Source: CAD feature listing. Evaluate the final solid. Frame: model axes, mm. Face numbers are marked on the shaded views. A direction names the side the tool comes from. Coordinates: 2 decimals unless noted, no trailing zeros. Order: outer loops, then holes, each group sorted by start corner. A loop starts at its lowest first (then second) coordinate and runs counter-clockwise, first axis right, second up. Notation, with made-up numbers: (84, 55) -> (103, 55) arc R19 cw to (103, 88) -> close; hole circle Ø7 at (73, 14.25). An arc over 180 degrees is marked (long way). Put each result on its own line as item: value.
from build123d import *

# Parameters (mm, degrees)
BOSS_EXTRUDE1_DEPTH      = 3
SKETCH4_R                = 2
CUT_EXTRUDE1_DEPTH       = 3
SKETCH5_R                = 3
CUT_EXTRUDE2_DEPTH       = 1
SKETCH6_R                = 1.5
CUT_EXTRUDE3_DEPTH       = 2
BOSS_EXTRUDE2_DEPTH      = 40
BOSS_EXTRUDE3_DEPTH      = 30
BOSS_EXTRUDE3_DEPTH_BACK = 30
SKETCH7_R                = 2
CUT_EXTRUDE5_REACH       = 83.646


with BuildPart() as part:
    # Sketch2 → Boss-Extrude1 (new body)
    with BuildSketch(Plane.XY):
        Polygon((33.535533906, -16.035533906), (3.535533906, -16.035533906), (0, -12.5), (0, 12.5), (3.535533906, 16.035533906), (23.535533906, 16.035533906), (56.464466094, 5.07852329), (60, 1.542989384), (60, -8.457010616), (56.464466094, -11.992544522), align=None)
    boss_extrude1 = extrude(amount=BOSS_EXTRUDE1_DEPTH)

    # Sketch4 → Cut-Extrude1 (cut)
    with BuildSketch(Plane(origin=(0, 0, 0), x_dir=(-1, 0, 0), z_dir=(0, 0, -1))):
        with Locations((-18, -1.035533906)):
            Circle(SKETCH4_R)
    cut_extrude1 = extrude(amount=-CUT_EXTRUDE1_DEPTH, mode=Mode.SUBTRACT)

    # Sketch5 → Cut-Extrude2 (cut)
    with BuildSketch(Plane(origin=(0, 0, 0), x_dir=(-1, 0, 0), z_dir=(0, 0, -1))):
        with Locations((-18, 6.964466094)):
            Circle(SKETCH5_R)
        with Locations((-10, -1.035533906)):
            Circle(SKETCH5_R)
        with Locations((-18, -9.035533906)):
            Circle(SKETCH5_R)
        with Locations((-26, -1.035533906)):
            Circle(SKETCH5_R)
    cut_extrude2 = extrude(amount=-CUT_EXTRUDE2_DEPTH, mode=Mode.SUBTRACT)

    # Sketch6 → Cut-Extrude3 (cut)
    with BuildSketch(Plane(origin=(0, 0, 1), x_dir=(-1, 0, 0), z_dir=(0, 0, -1))):
        with Locations((-18, 6.964466094)):
            Circle(SKETCH6_R)
        with Locations((-26, -1.035533906)):
            Circle(SKETCH6_R)
        with Locations((-10, -1.035533906)):
            Circle(SKETCH6_R)
        with Locations((-18, -9.035533906)):
            Circle(SKETCH6_R)
    cut_extrude3 = extrude(amount=-CUT_EXTRUDE3_DEPTH, mode=Mode.SUBTRACT)

    # Sketch3 → Boss-Extrude2 (add)
    with BuildSketch(Plane.XY.offset(3)):
        Polygon((8.69213043, 9.878421931), (7.795554958, 13.224487146), (4.449489743, 14.121062618), (2, 11.671572875), (2.896575472, 8.32550766), (6.242640687, 7.428932188), align=None)
        Polygon((36.226681597, -13.530158735), (37.411474128, -10.27496801), (35.184792531, -7.621312217), (31.773318403, -8.22284715), (30.588525872, -11.478037875), (32.815207469, -14.131693668), align=None)
        Polygon((36.846550019, 6.760383974), (36.24355834, 9.699159405), (33.397008321, 10.646341008), (31.153449981, 8.65474718), (31.75644166, 5.715971749), (34.602991679, 4.768790146), align=None)
    extrude(amount=BOSS_EXTRUDE2_DEPTH)

    # Mirror1: Boss-Extrude1, Cut-Extrude1, Cut-Extrude2, Cut-Extrude3 across plane
    add(boss_extrude1.mirror(Plane.XY.offset(23)))
    add(cut_extrude1.mirror(Plane.XY.offset(23)), mode=Mode.SUBTRACT)
    add(cut_extrude2.mirror(Plane.XY.offset(23)), mode=Mode.SUBTRACT)
    add(cut_extrude3.mirror(Plane.XY.offset(23)), mode=Mode.SUBTRACT)

    # Sketch7 → Boss-Extrude3 (add, two sides: drawn at the far end of the back side and taken through both)
    with BuildSketch(Plane.XY.offset(23).offset(-BOSS_EXTRUDE3_DEPTH_BACK)):
        with Locations((50, -3.457010616)):
            Circle(SKETCH7_R)
    extrude(amount=BOSS_EXTRUDE3_DEPTH + BOSS_EXTRUDE3_DEPTH_BACK)

    # Cut-Extrude5: up to this face of the body (flat: up to its plane)
    cut_extrude5_end = Plane(part.part.faces().sort_by_distance((18.535533906, -15.35519918, 46))[0])
    # Sketch9 → Cut-Extrude5 (cut, up to the picked face)
    with BuildSketch(Plane(origin=(0, 0, 0), x_dir=(-1, 0, 0), z_dir=(0, 0, -1)), mode=Mode.PRIVATE) as cut_extrude5_sk1:
        Polygon((0, -8.964466094), (-7.071067812, -16.035533906), (0, -16.035533906), align=None)
    cut_extrude5_tool1 = split(extrude(cut_extrude5_sk1.sketch, amount=-CUT_EXTRUDE5_REACH, mode=Mode.PRIVATE), bisect_by=cut_extrude5_end, keep=Keep.BOTH, mode=Mode.PRIVATE)
    add(cut_extrude5_tool1.solids().sort_by(Axis((2.357023, -13.678511, 0), (0, 0, 1)))[0], mode=Mode.SUBTRACT)


solid = part.part
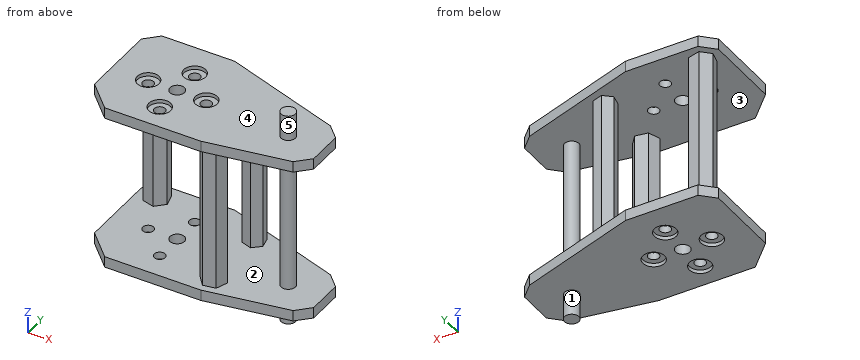
1. Cut plane C-C on x = 18. Count the separate pieces of the cut face and the enclosed holes in it, plus the area to 3 significant figures.
Numbers:
separate pieces: 8
enclosed holes: 0
area: 120 mm2
2. Pull-direction query (Z, two-part tool) for the marked faces 3, 4 and 5; classes: pulls with the +Z half, pulls with the -Z half, needs draft (parallel to the pull), parting line crosses it, or undercut.
Numbers:
face 3: undercut
face 4: pulls with the +Z half
face 5: needs draft
3. First-contact query: pin 1 (5 mm diameter, centred on x = 26, y = -1.04, fed in from -Z); pin 2 (5 mm diameter, centred on y = 5.5, z = -0.5, fed in from -X); pin 3 (1.5 mm diameter, centred on x = 20.5, y = -9, fed in from +Z); pin 4 (6.5 mm diameter, centred on x = 19, y = 7, fed in from -Z). Flat tips, straight axial feed; report the tip coordinate or a pass-through.
Numbers:
pin 1: stops at z = 1
pin 2: stops at x = 0
pin 3: stops at z = 46
pin 4: stops at z = 0
4. Ray query, line 1 along Y through (x, z) = (18, 43.45); line 2 along Y through (x, z) = (18, 45.75); line 3 along Z through (x, y) = (44, -2). Return the intervals inside material, ascending.
Numbers:
line 1: y = -16.04 to -10.54, -7.54 to -3.04, 0.96 to 5.46, 8.46 to 16.04
line 2: y = -16.04 to -12.04, -6.04 to -3.04, 0.96 to 3.96, 9.96 to 16.04
line 3: z = 0 to 3, 43 to 46
5. Cut plane D-D on z = -1. Output: boundary loops of the cut face in (x, y), plus the area to 3 significant figures.
Numbers:
outline: circle Ø4 at (50, -3.46)
area: 12.6 mm2
6. Cut plane A-A on x = 10. Output: boundary loops of the cut face in (y, z).
Numbers:
outline: (-16.04, 0) -> (-4.04, 0) -> (-4.04, 1) -> (-2.54, 1) -> (-2.54, 3) -> (-16.04, 3) -> close; (-16.04, 43) -> (-2.54, 43) -> (-2.54, 45) -> (-4.04, 45) -> (-4.04, 46) -> (-16.04, 46) -> close; (0.46, 1) -> (1.96, 1) -> (1.96, 0) -> (16.04, 0) -> (16.04, 3) -> (0.46, 3) -> close; (0.46, 43) -> (16.04, 43) -> (16.04, 46) -> (1.96, 46) -> (1.96, 45) -> (0.46, 45) -> close
7. Set-up query: the marked faces 1 and 2. Return all of +Z, -Z, +X, -X, +Y, -Y with unobstructed straight access to the full face (end or side cutting, diameter ignored); none if empty.
Numbers:
face 1: -Z
face 2: none
8. Cut plane B-B on z = 17.5. Output: boundary loops of the cut face in (x, y), plus the area to 3 significant figures.
Numbers:
outline: (2, 11.67) -> (2.9, 8.33) -> (6.24, 7.43) -> (8.69, 9.88) -> (7.8, 13.22) -> (4.45, 14.12) -> close; (30.59, -11.48) -> (32.82, -14.13) -> (36.23, -13.53) -> (37.41, -10.27) -> (35.18, -7.62) -> (31.77, -8.22) -> close; (31.15, 8.65) -> (31.76, 5.72) -> (34.6, 4.77) -> (36.85, 6.76) -> (36.24, 9.7) -> (33.4, 10.65) -> close; circle Ø4 at (50, -3.46)
area: 98.3 mm2
